Check sheet for the modelled part. Datum: model origin and axes. Units: mm. Face numbers are marked on the shaded views. A direction names the side the tool comes from. Round coordinates to 2 decimals unless told otherwise and drop trailing zeros. Loops run counter-clockwise (first coordinate to the right, second up) from the corner with the lowest first, then second, coordinate; pieces in that order, holes last. Notation, with made-up numbers: (-35, 80.5) -> (17, 80.5) arc R23 ccw to (17, 95.5) -> close; hole circle Ø11 at (-31.5, 60.25). An arc over 180 degrees is marked (long way). One line per question, with ' | ' between items.
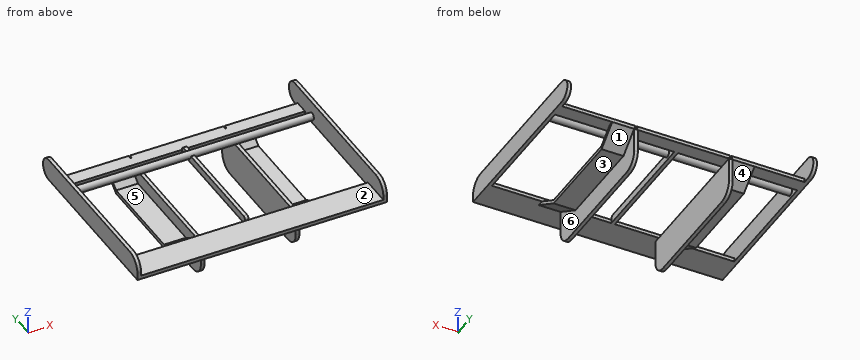
```python
from build123d import *

# Parameters (mm, degrees)
SKETCH1_W                       = 25
SKETCH1_H                       = 264
BOSS_EXTRUDE1_DEPTH             = 958
BOSS_EXTRUDE2_DEPTH             = 150
SKETCH3_W                       = 1660
SKETCH3_H                       = 95
SKETCH3_H_2                     = 200
BOSS_EXTRUDE3_DEPTH             = 25
SKETCH4_W                       = 150
SKETCH4_H                       = 1230
BOSS_EXTRUDE4_DEPTH             = 25
BOSS_EXTRUDE5_REACH             = 1435.453
SKETCH5_R                       = 25
BOSS_EXTRUDE5_DIRECTION_2_REACH = 1435.453
BOSS_EXTRUDE6_REACH             = 1362.836
SKETCH6_W                       = 25
SKETCH6_H                       = 50
FILLET1_RADIUS                  = 75
FILLET1_LENGTH                  = 25
FILLET2_RADIUS                  = 75
FILLET2_LENGTH                  = 25
FILLET3_R                       = 100
FILLET4_R                       = 100
FILLET5_R                       = 100
FILLET6_R                       = 100
FILLET7_R                       = 20
FILLET8_R                       = 20
FILLET9_R                       = 100
FILLET10_R                      = 100
CUT_EXTRUDE5_DEPTH              = 25


with BuildPart() as part:
    # Sketch1 → Boss-Extrude1 (new body)
    with BuildSketch(Plane(origin=(0, 0, 0), x_dir=(1, 0, 0), z_dir=(0, 1, 0))):
        with Locations((325, 0)):
            Rectangle(SKETCH1_W, SKETCH1_H)
    extrude(amount=-BOSS_EXTRUDE1_DEPTH)

    # Sketch2 → Boss-Extrude2 (add)
    with BuildSketch(Plane(origin=(337.5, 0, 0), x_dir=(0, 0, -1), z_dir=(1, 0, 0))):
        Polygon((-43, -139.55), (-43, -763.99), (-132, -915.453947368), (-132, -958), (-18, -763.99), (-18, -139.55), (-132, 0), (-132, -30.603070175), align=None)
    extrude(amount=BOSS_EXTRUDE2_DEPTH)


with BuildPart() as body_2:
    # Mirror2: mirrored copy
    add(part.part.mirror(Plane(origin=(0, 0, 0), x_dir=(0, 0, 1), z_dir=(1, 0, 0))))


with BuildPart() as part_1:
    add(part.part)

    add(body_2.part)  # Boss-Extrude3 merges body 2
    # Sketch3 → Boss-Extrude3 (add)
    with BuildSketch(Plane.XY.offset(132)):
        with Locations((0, -47.5)):
            Rectangle(SKETCH3_W, SKETCH3_H)
        with Locations((0, -1015.453947368)):
            Rectangle(SKETCH3_W, SKETCH3_H_2)
    extrude(amount=BOSS_EXTRUDE3_DEPTH)

    # Sketch4 → Boss-Extrude4 (add)
    with BuildSketch(Plane(origin=(830, 0, 0), x_dir=(0, 0, -1), z_dir=(1, 0, 0))):
        with Locations((-207, -500.453947368)):
            Rectangle(SKETCH4_W, SKETCH4_H)
    boss_extrude4 = extrude(amount=BOSS_EXTRUDE4_DEPTH)

    # Mirror3: Boss-Extrude4 across plane
    add(boss_extrude4.mirror(Plane(origin=(0, 0, 0), x_dir=(0, 0, 1), z_dir=(1, 0, 0))))

    # Sketch5 → Boss-Extrude5 (add, up to next)
    with BuildSketch(Plane(origin=(0, 0, 0), x_dir=(0, 0, -1), z_dir=(1, 0, 0)), mode=Mode.PRIVATE) as boss_extrude5_sk1:
        with Locations((-179.2, -185.96)):
            Circle(SKETCH5_R)
    boss_extrude5_tool1 = extrude(boss_extrude5_sk1.sketch, amount=BOSS_EXTRUDE5_REACH, mode=Mode.PRIVATE) - part_1.part
    add(boss_extrude5_tool1.solids().sort_by_distance((0, -185.96, 179.2))[0])

    # Sketch5 → Boss-Extrude5 direction 2 (add, up to next)
    with BuildSketch(Plane(origin=(0, 0, 0), x_dir=(0, 0, -1), z_dir=(1, 0, 0)), mode=Mode.PRIVATE) as boss_extrude5_direction_2_sk1:
        with Locations((-179.2, -185.96)):
            Circle(SKETCH5_R)
    boss_extrude5_direction_2_tool1 = extrude(boss_extrude5_direction_2_sk1.sketch, amount=-BOSS_EXTRUDE5_DIRECTION_2_REACH, mode=Mode.PRIVATE) - part_1.part
    add(boss_extrude5_direction_2_tool1.solids().sort_by_distance((0, -185.96, 179.2))[0])

    # Boss-Extrude6: up to this face of the body (flat: up to its plane)
    boss_extrude6_end = Plane(part_1.part.faces().sort_by_distance((0, -915.453947368, 144.5))[0])
    # Sketch6 → Boss-Extrude6 (add, up to the picked face)
    with BuildSketch(Plane.XZ.offset(95), mode=Mode.PRIVATE) as boss_extrude6_sk1:
        with Locations((0, 157)):
            Rectangle(SKETCH6_W, SKETCH6_H)
    boss_extrude6_tool1 = split(extrude(boss_extrude6_sk1.sketch, amount=BOSS_EXTRUDE6_REACH, mode=Mode.PRIVATE), bisect_by=boss_extrude6_end, keep=Keep.BOTH, mode=Mode.PRIVATE)
    add(boss_extrude6_tool1.solids().sort_by(Axis((0, -95, 157), (0, -1, 0)))[0])

    # Fillet1: full round fillet: the end face becomes a half cylinder, R = half its width
    fillet1_face = Plane((842.5, 114.546052632, 207), x_dir=(-1, 0, 0), z_dir=(0, 1, 0))  # on the end face: x along it, z out of the body
    fillet1_slab = fillet1_face.offset(-FILLET1_RADIUS / 2) * Box(FILLET1_LENGTH, 2 * FILLET1_RADIUS, FILLET1_RADIUS, mode=Mode.PRIVATE)  # the body's end, R deep
    fillet1_round = Plane((842.5, 39.546052632, 207), x_dir=(0, 1, 0), z_dir=(-1, 0, 0)) * Cylinder(FILLET1_RADIUS, FILLET1_LENGTH, mode=Mode.PRIVATE)  # its axis R under the face
    add(fillet1_slab - fillet1_round, mode=Mode.SUBTRACT)

    # Fillet2: full round fillet: the end face becomes a half cylinder, R = half its width
    fillet2_face = Plane((-842.5, 114.546052632, 207), x_dir=(-1, 0, 0), z_dir=(0, 1, 0))  # on the end face: x along it, z out of the body
    fillet2_slab = fillet2_face.offset(-FILLET2_RADIUS / 2) * Box(FILLET2_LENGTH, 2 * FILLET2_RADIUS, FILLET2_RADIUS, mode=Mode.PRIVATE)  # the body's end, R deep
    fillet2_round = Plane((-842.5, 39.546052632, 207), x_dir=(0, 1, 0), z_dir=(-1, 0, 0)) * Cylinder(FILLET2_RADIUS, FILLET2_LENGTH, mode=Mode.PRIVATE)  # its axis R under the face
    add(fillet2_slab - fillet2_round, mode=Mode.SUBTRACT)

    # Fillet3
    fillet3_edges = [part_1.edges().sort_by_distance(p)[0] for p in [
        (-325, 0, -132),
    ]]
    fillet(fillet3_edges, radius=FILLET3_R)

    # Fillet4
    fillet4_edges = [part_1.edges().sort_by_distance(p)[0] for p in [
        (325, 0, -132),
    ]]
    fillet(fillet4_edges, radius=FILLET4_R)

    # Fillet5
    fillet5_edges = [part_1.edges().sort_by_distance(p)[0] for p in [
        (325, -958, -132),
    ]]
    fillet(fillet5_edges, radius=FILLET5_R)

    # Fillet6
    fillet6_edges = [part_1.edges().sort_by_distance(p)[0] for p in [
        (-325, -958, -132),
    ]]
    fillet(fillet6_edges, radius=FILLET6_R)

    # Fillet7
    fillet7_edges = [part_1.edges().sort_by_distance(p)[0] for p in [
        (0, -95, 182),
    ]]
    fillet(fillet7_edges, radius=FILLET7_R)

    # Fillet8
    fillet8_edges = [part_1.edges().sort_by_distance(p)[0] for p in [
        (0, -915.453947368, 182),
    ]]
    fillet(fillet8_edges, radius=FILLET8_R)

    # Fillet9
    fillet9_edges = [part_1.edges().sort_by_distance(p)[0] for p in [
        (842.5, -1115.453947368, 282),
    ]]
    fillet(fillet9_edges, radius=FILLET9_R)

    # Fillet10
    fillet10_edges = [part_1.edges().sort_by_distance(p)[0] for p in [
        (-842.5, -1115.453947368, 282),
    ]]
    fillet(fillet10_edges, radius=FILLET10_R)

    # Sketch7 → Cut-Extrude5 (cut)
    with BuildSketch(Plane(origin=(0, 0, 0), x_dir=(1, 0, 0), z_dir=(0, 1, 0))):
        Polygon((337, -132), (313, -132), (321, -157), (329, -157), align=None)
    cut_extrude5 = extrude(amount=-CUT_EXTRUDE5_DEPTH, mode=Mode.SUBTRACT)

    # Mirror4: Cut-Extrude5 across plane
    add(cut_extrude5.mirror(Plane(origin=(0, 0, 0), x_dir=(0, 0, 1), z_dir=(1, 0, 0))), mode=Mode.SUBTRACT)


solid = part_1.part
```
(1) Mould release check, pull along Y, two halves, no side actions. Record for the marked faces 4, 5 and 6: +Y half, -Y half, draft (parallel to the pull), parting line (faces both ways), or undercut.
Answer:
face 4: +Y half | face 5: undercut | face 6: draft
(2) Sectioned sample at C-C, the plane x = -427.5. Record the cut outline in (y, z), and give its area (3 significant figures).
Answer:
outline: (-1115.45, 132) -> (-958, 132) -> (-763.99, 18) -> (-139.55, 18) -> (0, 132) -> (0, 157) -> (-95, 157) -> (-95, 132) -> (-30.6, 132) -> (-139.55, 43) -> (-763.99, 43) -> (-915.45, 132) -> (-915.45, 157) -> (-1115.45, 157) -> close; circle Ø50 at (-185.96, 179.2) | area: 32,400 mm2
(3) Sectioned sample at D-D, the plane y = -558.5. Record the cut outline in (x, z), and give its area (4 significant figures).
Answer:
outline: (-855, 132) -> (-830, 132) -> (-830, 282) -> (-855, 282) -> close; (-487.5, 18) -> (-337.5, 18) -> (-337.5, -132) -> (-312.5, -132) -> (-312.5, 132) -> (-337.5, 132) -> (-337.5, 43) -> (-487.5, 43) -> close; (-12.5, 132) -> (12.5, 132) -> (12.5, 182) -> (-12.5, 182) -> close; (312.5, -132) -> (337.5, -132) -> (337.5, 18) -> (487.5, 18) -> (487.5, 43) -> (337.5, 43) -> (337.5, 132) -> (312.5, 132) -> close; (830, 132) -> (855, 132) -> (855, 282) -> (830, 282) -> close | area: 29,450 mm2
(4) Scan lines: probe 1 along X at (y, z) = (-365, 135.5); probe 2 along X at (y, z) = (-642.5, 86.5); probe 3 along Y at (x, z) = (375, 136). Record each from-to range of solid material in increasing order.
Answer:
probe 1: x = -855 to -830, -12.5 to 12.5, 830 to 855 | probe 2: x = -337.5 to -312.5, 312.5 to 337.5 | probe 3: y = -1115.45 to -915.45, -95 to 0
(5) Set-up check for the marked faces 1, 2 and 3: record each of +Z, -Z, +X, -X, +Y, -Y from which the full face is reachable in a straight line by a thin tool's end or side.
Answer:
face 1: -Z, +X, +Y | face 2: +Z, -Y | face 3: -Z, +X, +Y, -Y
(6) Sectioned sample at A-A, the plane y = -185.96. Count the separate pieces of the cut face and the enclosed holes in it, and give its area (3 significant figures).
Answer:
separate pieces: 3 | enclosed holes: 0 | area: 112,000 mm2
(7) Sectioned sample at B-B, the plane x = -159. Record the cut outline in (y, z), and give its area (3 significant figures).
Answer:
outline: (-1115.45, 132) -> (-915.45, 132) -> (-915.45, 157) -> (-1115.45, 157) -> close; circle Ø50 at (-185.96, 179.2); (-95, 132) -> (0, 132) -> (0, 157) -> (-95, 157) -> close | area: 9,340 mm2
(8) Go/stop test with flat-tipped pins: pin 1 (7 mm diameter, centred on x = -320.5, y = -8, fed in from +Z); pin 2 (1.5 mm diameter, centred on x = 348, z = 131, fed in from +Y); pin 3 (2.5 mm diameter, centred on x = -4.5, z = 159, fed in from -Y). Record where each tip stops, or that it passes through.
Answer:
pin 1: stops at z = 157 | pin 2: stops at y = -0.31 | pin 3: stops at y = -915.45
